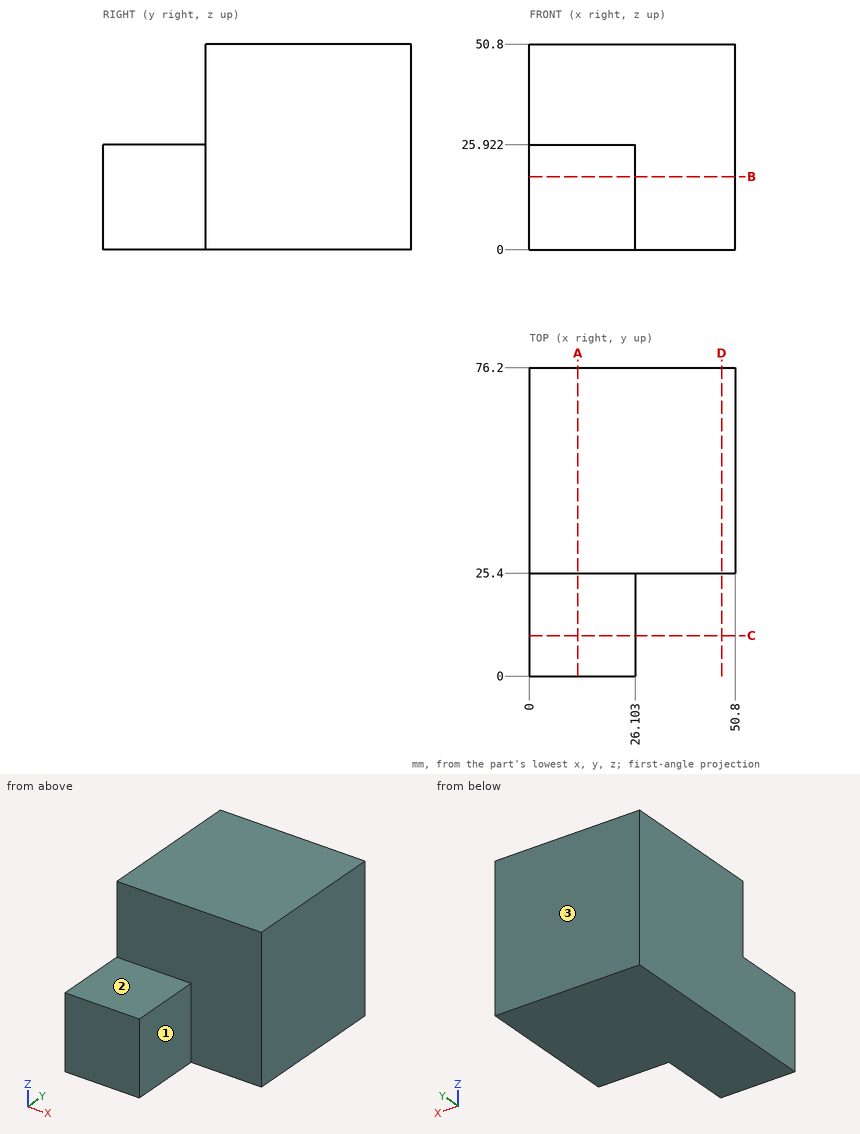
Verification items for this drawing (mm, ordinates from the low corner). A direction names the side the tool comes from. Round coordinates to 2 decimals unless told otherwise and drop trailing zeros. Order: outer loops, then holes, each group sorted by start corner. A loop starts at its lowest first (then second) coordinate and runs counter-clockwise, first axis right, second up. Notation, with made-up numbers: (81, 53.25) - (137, 53.25) arc R23 cw to (137, 91.25) - close; hole circle Ø6 at (47, -33). An arc over 180 degrees is marked (long way). Use CSV: the item, a comma, the result in double quotes. Start each with the question number.
1) Section check D-D, the plane x = 47.5. Record the cut outline in (y, z), plus the area to 3 significant figures.
2) Access from +Z, -Z, +X, -X, +Y, -Y to the whole of each face (thin tool, end or side, straight path). Record for the marked faces 1, 2 and 3.
3) Thickness scan on L1, parallel to X at y = 22.5, z = 23; L2, parallel to Y at x = 5.5, z = 42.5; L3, parallel to Z at x = 10.5, y = 9. Record the ranges inside material, lowest first.
4) Section check B-B, the plane z = 18. Record the cut outline in (x, y).
5) Section check A-A, the plane x = 12. Record the cut outline in (y, z).
6) Go/stop test with flat-tipped pins: P1, Ø4, axis at y = 59.5, z = 6, coming from the -X side; P2, Ø2, axis at y = 16.5, z = 25.5, coming from the +X side. Record where each tip stops, or that it passes through.
7) Section check C-C, the plane y = 10. Record the cut outline in (x, z), plus the area to 3 significant figures.
Answers:
1,outline,"(25.4, 0) - (76.2, 0) - (76.2, 50.8) - (25.4, 50.8) - close"
1,area,"2,580 mm²"
2,face 1,"+Z, -Z, +X, -Y"
2,face 2,"+Z, +X, -X, -Y"
2,face 3,"+Z, -Z, +X, -X, +Y"
3,L1,"x = 0 to 26.1"
3,L2,"y = 25.4 to 76.2"
3,L3,"z = 0 to 25.92"
4,outline,"(0, 0) - (26.1, 0) - (26.1, 25.4) - (50.8, 25.4) - (50.8, 76.2) - (0, 76.2) - close"
5,outline,"(0, 0) - (76.2, 0) - (76.2, 50.8) - (25.4, 50.8) - (25.4, 25.92) - (0, 25.92) - close"
6,P1,"stops at x = 0"
6,P2,"stops at x = 26.1"
7,outline,"(0, 0) - (26.1, 0) - (26.1, 25.92) - (0, 25.92) - close"
7,area,"677 mm²"
